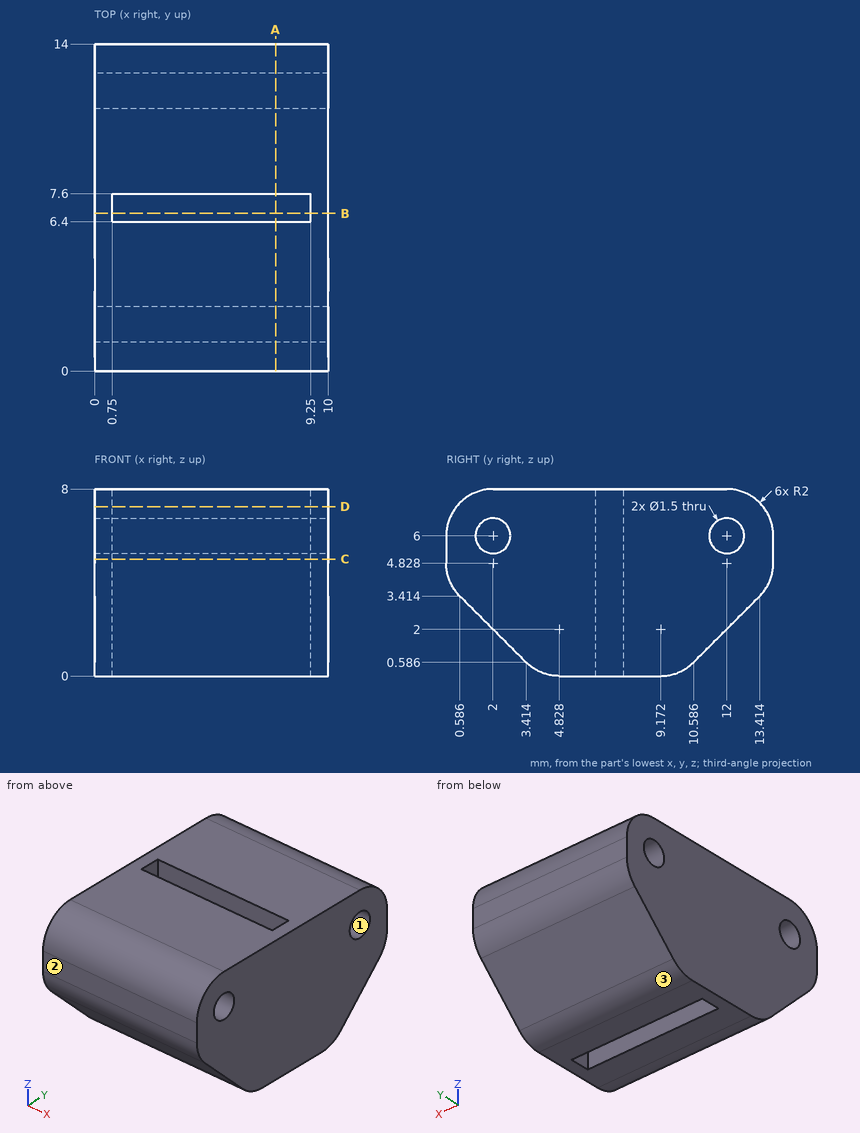
Check sheet for the drawn part. Datum: minimum x, y, z corner. Units: mm. Give positions to 0.01 mm unless a question says otherwise; leave off trailing zeros. Write each loop counter-clockwise with the first axis right and the second up, starting at its lowest first coordinate (ties: lowest second). Pieces come first, ordered by that corner, then holes.
(1) Gauge pin test, flat end, axial feed: pin 1 (1 mm diameter, centred on y = 7, z = 6, fed in from -X). Record the tip position at first contact, or that the pin passes through.
(2) Cross-section at B-B (y = 6.75). Enter the section's corners in (x, z), plus the area to 3 significant figures.
(3) Cross-section at C-C (z = 5). Enter the section's corners in (x, y), plus the area to 3 significant figures.
(4) Material ranges on line 1 (Y direction, x = 6.75, z = 6.5) (1 decimal); line 2 (X direction, y = 7.25, z = 7.5); line 3 (Z direction, x = 4, y = 9.25), recorded low to high.
(5) Cross-section at A-A (x = 7.75). State how many separate pieces and enclosed holes the cut face has.
(6) Cross-section at D-D (z = 7.25). Enter the section's corners in (x, y).
(7) Mould release check, pull along Z, two halves, no side actions. Record for the marked faces 1, 2 and 3: +Z half, -Z half, draft (parallel to the pull), parting line (faces both ways), or undercut.
Worked out:
1. pin 1: stops at x = 0
2. outline: (0, 0) - (0.75, 0) - (0.75, 8) - (0, 8) - close; (9.25, 0) - (10, 0) - (10, 8) - (9.25, 8) - close
2. area: 12.0 mm2
3. outline: (0, 0) - (10, 0) - (10, 14) - (0, 14) - close; hole (0.75, 6.4) - (9.25, 6.4) - (9.25, 7.6) - (0.75, 7.6) - close
3. area: 130 mm2
4. line 1: y = 0.1 to 1.4, 2.6 to 6.4, 7.6 to 11.4, 12.6 to 13.9
4. line 2: x = 0 to 0.75, 9.25 to 10
4. line 3: z = 0 to 8
5. separate pieces: 2
5. enclosed holes: 2
6. outline: (0, 0.44) - (10, 0.44) - (10, 13.56) - (0, 13.56) - close; hole (0.75, 6.4) - (9.25, 6.4) - (9.25, 7.6) - (0.75, 7.6) - close
7. face 1: undercut
7. face 2: draft
7. face 3: -Z half
